Read the model definition and answer for the solid it produces. Units are mm, in the model's axes. A direction names the side the tool comes from. Coordinates: 2 decimals unless noted, no trailing zeros. Write each loop counter-clockwise with the first axis right and the second up, starting at its lowest first coordinate (ties: lowest second). Pieces come first, ordered by that corner, then holes. Notation, with made-up numbers: M 83.5,-0.5 L 112.5,-0.5 A17 cw 112.5,17.5 Z; hole C 62.5,79 d7. An arc over 180 degrees is marked long. Use a Markdown table: item, result. Add a question column.
from build123d import *

# Parameters (mm, degrees)
ESTRUSIONE_ESTRUSIONE1_DEPTH                         = 30
SCHIZZO2_R                                           = 9.999999999999993
TAGLIO_ESTRUSIONE1_DEPTH                             = 18
FORO_LAMATO_PER_VITE_M6_A_TESTA_CILINDRI_D           = 6.6
FORO_LAMATO_PER_VITE_M6_A_TESTA_CILINDRI_DEPTH       = 80
FORO_LAMATO_PER_VITE_M6_A_TESTA_CILINDRI_CBORE_D     = 15
FORO_LAMATO_PER_VITE_M6_A_TESTA_CILINDRI_CBORE_DEPTH = 5
FORO_LAMATO_PER_VITE_M6_A_TESTA_CILINDRI_TIP         = 1.982840042790949
SMUSSO1_SIZE                                         = 2
SCHIZZO6_R                                           = 6.000000000000001
TAGLIO_ESTRUSIONE2_DEPTH                             = 3


with BuildPart() as part:
    # Schizzo1 → Estrusione-Estrusione1 (new body)
    with BuildSketch(Plane(origin=(0, 0, 0), x_dir=(1, 0, 0), z_dir=(0, 1, 0))):
        Polygon((0, 0), (-45, -6.12e-15), (-45, 24.999999999999993), (0, 25.000000000000004), align=None)
    extrude(amount=ESTRUSIONE_ESTRUSIONE1_DEPTH)

    # Schizzo2 → Taglio-Estrusione1 (cut)
    with BuildSketch(Plane(origin=(-5.78e-15, 0, -25.000000000000004), x_dir=(-1, 0, 2.1e-16), z_dir=(-2.1e-16, 0, -1))):
        with Locations((22.499999999999993, 18)):
            Circle(SCHIZZO2_R)
    extrude(amount=-TAGLIO_ESTRUSIONE1_DEPTH, mode=Mode.SUBTRACT)

    # Foro lamato per Vite M6 a testa cilindrica-1
    with Locations(Plane(origin=(0, 0, 0), x_dir=(0, 0, -1), z_dir=(1, 0, 0))):
        with Locations((15, 18)):
            CounterBoreHole(FORO_LAMATO_PER_VITE_M6_A_TESTA_CILINDRI_D / 2, FORO_LAMATO_PER_VITE_M6_A_TESTA_CILINDRI_CBORE_D / 2, FORO_LAMATO_PER_VITE_M6_A_TESTA_CILINDRI_CBORE_DEPTH, depth=FORO_LAMATO_PER_VITE_M6_A_TESTA_CILINDRI_DEPTH)
            with Locations((0, 0, -(FORO_LAMATO_PER_VITE_M6_A_TESTA_CILINDRI_DEPTH + FORO_LAMATO_PER_VITE_M6_A_TESTA_CILINDRI_TIP / 2))):  # 118° drill point
                Cone(0, FORO_LAMATO_PER_VITE_M6_A_TESTA_CILINDRI_D / 2, FORO_LAMATO_PER_VITE_M6_A_TESTA_CILINDRI_TIP, mode=Mode.SUBTRACT)

    # Smusso1
    smusso1_edges = [part.edges().sort_by_distance(p)[0] for p in [
        (-45, 30, -12.499999999999995),
        (-22.5, 30, 3.06e-15),
        (0, 30, -12.500000000000002),
        (-22.5, 0, 3.06e-15),
        (-45, 0, -12.499999999999995),
        (-22.5, 0, -25),
        (0, 0, -12.500000000000002),
        (0, 15, 0),
        (-45, 15, 6.12e-15),
        (-45, 15, -24.999999999999993),
        (0, 15, -25.000000000000004),
        (-22.5, 30, -25),
    ]]
    chamfer(smusso1_edges, length=SMUSSO1_SIZE)

    # Schizzo6 → Taglio-Estrusione2 (cut)
    with BuildSketch(Plane.ZY.offset(45)):
        with Locations((-15.000000000000005, 18)):
            Circle(SCHIZZO6_R)
    extrude(amount=-TAGLIO_ESTRUSIONE2_DEPTH, mode=Mode.SUBTRACT)


solid = part.part
Item 1: Find section D-D on z = -21.5. Give the vertices of the cut face in (x, y), then the cut area to 3 significant figures.
Item 2: Consider probe 1 along Y at (x, z) = (-39, -15); probe 2 along Z at (x, y) = (-35, 18); probe 3 along Y at (x, z) = (-22.5, -11). Determine where each line is inside the solid, lowest interval first.
Item 3: Find section B-B on y = 18. Give the vertices of the cut face in (x, z).
Item 4: Determine the mould class of faces 4 (the cylindrical face through (-37.04, 15.992, -17.619)), 5 (the flat face through (-1.2, 28.6, -1.4)), 6 (the cylindrical face through (-31.737, 14.17, -16.126)), 7 (the flat face through (-1, 1, -13)) for opening direction Y: pulls with the +Y half, pulls with the -Y half, needs draft (parallel to the pull), parting line crosses it, or undercut.
Item 5: Find section A-A on z = -15. Give the vertices of the cut face in (x, y).
Item 6: Find section C-C on x = -40. Give the vertices of the cut face in (y, z).
Item 7: Each of these flat-tipped pins is pushed along its axis until it touches: pin 1 (2 mm diameter, centred on y = 14, z = -18.5, fed in from +X); pin 2 (8.5 mm diameter, centred on y = 18, z = -15, fed in from -X). Where does it stop, or does it pass through?
Item 8: For faces 1 (the flat face through (-1.2, 1.4, -1.4)), 2 (the cylindrical face through (-2.465, 25.436, -14.024)), 3 (the flat face through (-22, 18, -7)), determine the directions among +Z, -Z, +X, -X, +Y, -Y from which every point of the face is accessible in a straight line to the end or side of a thin tool.
Geometry says:
| question | item | result |
|---|---|---|
| 1 | outline | M -45,2 L -43,0 L -2,0 L 0,2 L 0,14.26 L -5,14.26 L -5,21.74 L 0,21.74 L 0,28 L -2,30 L -43,30 L -45,28 Z; hole C -22.5,18 d20 |
| 1 | area | 990 mm2 |
| 2 | probe 1 | y = 0 to 14.7, 21.3 to 30 |
| 2 | probe 2 | z = -25 to -18.3, -11.7 to 0 |
| 2 | probe 3 | y = 0 to 8, 28 to 30 |
| 3 | outline | M -45,-23 L -43,-25 L -32.5,-25 L -32.5,-18.3 L -42,-18.3 L -42,-21 L -45,-21 Z; M -45,-9 L -42,-9 L -42,-11.7 L -32.5,-11.7 L -32.5,-7 L -12.5,-7 L -12.5,-11.7 L -5,-11.7 L -5,-7.5 L 0,-7.5 L 0,-2 L -2,0 L -43,0 L -45,-2 Z; M -12.5,-25 L -2,-25 L 0,-23 L 0,-22.5 L -5,-22.5 L -5,-18.3 L -12.5,-18.3 Z |
| 4 | face 4 | undercut |
| 4 | face 5 | pulls with the +Y half |
| 4 | face 6 | undercut |
| 4 | face 7 | pulls with the -Y half |
| 5 | outline | M -45,2 L -43,0 L -2,0 L 0,2 L 0,10.5 L -5,10.5 L -5,14.7 L -13.06,14.7 A10 cw -31.94,14.7 L -42,14.7 L -42,12 L -45,12 Z; M -45,24 L -42,24 L -42,21.3 L -31.94,21.3 A10 cw -13.06,21.3 L -5,21.3 L -5,25.5 L 0,25.5 L 0,28 L -2,30 L -43,30 L -45,28 Z |
| 6 | outline | M 0,-23 L 2,-25 L 28,-25 L 30,-23 L 30,-2 L 28,0 L 2,0 L 0,-2 Z; hole C 18,-15 d6.6 |
| 7 | pin 1 | stops at x = -5 |
| 7 | pin 2 | stops at x = -42 |
| 8 | face 1 | +Z, +X, -Y |
| 8 | face 2 | +X |
| 8 | face 3 | -Z |
